For this review, take the finished solid that the model builds, in its own axes (mm). Face numbers are marked on the shaded views. Coordinates: 2 decimals unless noted, no trailing zeros. Loops run counter-clockwise (first coordinate to the right, second up) from the corner with the lowest first, then second, coordinate; pieces in that order, holes last. Notation, with made-up numbers: M 40,-15.75 L 87,-15.75 A23 cw 87,0.25 Z; hole C 60,41.5 d4. An arc over 180 degrees is marked long. Write item = value, one per line.
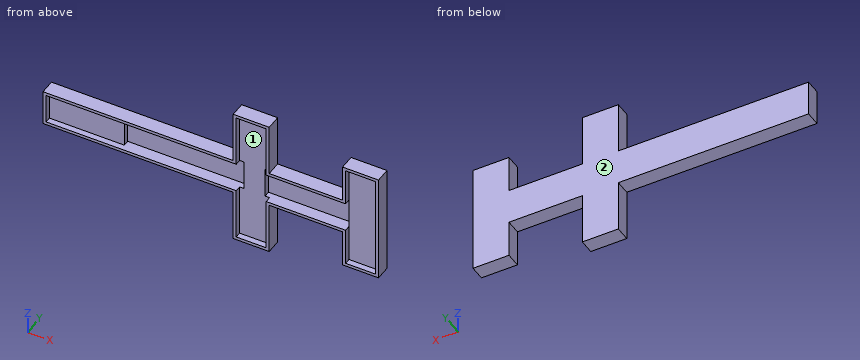
from build123d import *

# Parameters (mm, degrees)
SKETCH_3_W           = 10
SKETCH_3_H           = 35
SKETCH_3_W_2         = 26.5
SKETCH_3_H_2         = 10
SKETCH_3_W_3         = 38.5
SKETCH_3_W_4         = 25
EXTRUDE_1_DEPTH      = 1
EXTRUDE_2_DEPTH      = 4
EXTRUDE_2_DEPTH_BACK = 1
SKETCH_5_W           = 25
SKETCH_5_H           = 10
SKETCH_5_W_2         = 10
SKETCH_5_H_2         = 35
EXTRUDE_3_DEPTH      = 2


with BuildPart() as part:
    # 草图3 → 凸台-拉伸1 (new body)
    with BuildSketch(Plane(origin=(0, 0, 0), x_dir=(1, 0, 0), z_dir=(0, 1, 0))):
        with Locations((19, 0)):
            Rectangle(SKETCH_3_W, SKETCH_3_H)
        with Locations((0.75, 0)):
            Rectangle(SKETCH_3_W_2, SKETCH_3_H_2)
        Polygon((-12.5, -5), (-12.5, 5), (-12.5, 22.5), (-22.5, 22.5), (-22.5, 5), (-22.5, -5), (-22.5, -22.5), (-12.5, -22.5), align=None)
        with Locations((-41.75, 0)):
            Rectangle(SKETCH_3_W_3, SKETCH_3_H_2)
        with Locations((-73.5, 0)):
            Rectangle(SKETCH_3_W_4, SKETCH_3_H_2)
    extrude(amount=EXTRUDE_1_DEPTH)

    # 草图4 → 凸台-拉伸2 (add, two sides)
    with BuildSketch(Plane.XZ) as extrude_2_sk:
        Polygon((13, -18.5), (25, -18.5), (25, 18.5), (13, 18.5), (13, 6), (-11.5, 6), (-11.5, 23.5), (-23.5, 23.5), (-23.5, 6), (-87, 6), (-87, -6), (-23.5, -6), (-23.5, -23.5), (-11.5, -23.5), (-11.5, -6), (13, -6), align=None)
        Polygon((14, -17.5), (24, -17.5), (24, 17.5), (14, 17.5), (14, 5), (-12.5, 5), (-12.5, 22.5), (-22.5, 22.5), (-22.5, 5), (-86, 5), (-86, -5), (-22.5, -5), (-22.5, -22.5), (-12.5, -22.5), (-12.5, -5), (14, -5), align=None, mode=Mode.SUBTRACT)
    extrude(amount=EXTRUDE_2_DEPTH)
    extrude(extrude_2_sk.sketch, amount=-EXTRUDE_2_DEPTH_BACK)

    # 草图5 → 凸台-拉伸3 (add)
    with BuildSketch(Plane.XZ):
        Polygon((-22.5, 22.5), (-22.5, 5), (-21, 5), (-21, -5), (-22.5, -5), (-22.5, -22.5), (-12.5, -22.5), (-12.5, -5), (-14, -5), (-14, 5), (-12.5, 5), (-12.5, 22.5), align=None)
        with Locations((-73.5, 0)):
            Rectangle(SKETCH_5_W, SKETCH_5_H)
        with Locations((19, 0)):
            Rectangle(SKETCH_5_W_2, SKETCH_5_H_2)
    extrude(amount=EXTRUDE_3_DEPTH)


solid = part.part
Q1. Add section D-D (z = 20). Write out the cut boundary in (x, y).
Solved:
outline = M -23.5,-4 L -22.5,-4 L -22.5,-2 L -12.5,-2 L -12.5,-4 L -11.5,-4 L -11.5,1 L -23.5,1 Z
Q2. For pin 1 Ø2 at (x, y) = (-4.5, -1.5) entering from +Z; pin 2 Ø1.5 at (y, z) = (0, -14.5) entering from -X; pin 3 Ø2 at (x, z) = (10.5, 12.5) entering from +Y; pin 4 Ø1.6 at (x, y) = (19, -3) entering from +Z, all flat-tipped, find the tip position at first contact; note any pin that passes through.
Solved:
pin_1 = 6
pin_2 = -23.5
pin_3 = through
pin_4 = 18.5
Q3. For line 1 along X through (y, z) = (-1.3, -2); line 2 along X through (y, z) = (-2.8, 11); line 3 along X through (y, z) = (-1.95, -9), list the stretches that pass through material, from the lowest coordinate up.
Solved:
line_1 = -87 to -61, -21 to -14, 14 to 25
line_2 = -23.5 to -22.5, -12.5 to -11.5, 13 to 14, 24 to 25
line_3 = -23.5 to -11.5, 13 to 25
Q4. Draft analysis for pull direction Z (two halves, no side actions). For the marked faces 1 and 2, state which applies: +Z half, -Z half, draft (parallel to the pull), parting line (faces both ways), or undercut.
Solved:
face_1 = undercut
face_2 = draft
Q5. Add section A-A (z = 14.5). Write out the cut boundary in (x, y), and give its area (3 significant figures).
Solved:
outline = M -23.5,-4 L -22.5,-4 L -22.5,-2 L -12.5,-2 L -12.5,-4 L -11.5,-4 L -11.5,1 L -23.5,1 Z; M 13,-4 L 14,-4 L 14,-2 L 24,-2 L 24,-4 L 25,-4 L 25,1 L 13,1 Z
area = 80.0 mm²
Q6. Add section C-C (x = -65). Write out the cut boundary in (y, z), and give its area (3 significant figures).
Solved:
outline = M -4,-6 L 1,-6 L 1,6 L -4,6 L -4,5 L -2,5 L -2,-5 L -4,-5 Z
area = 40.0 mm²
